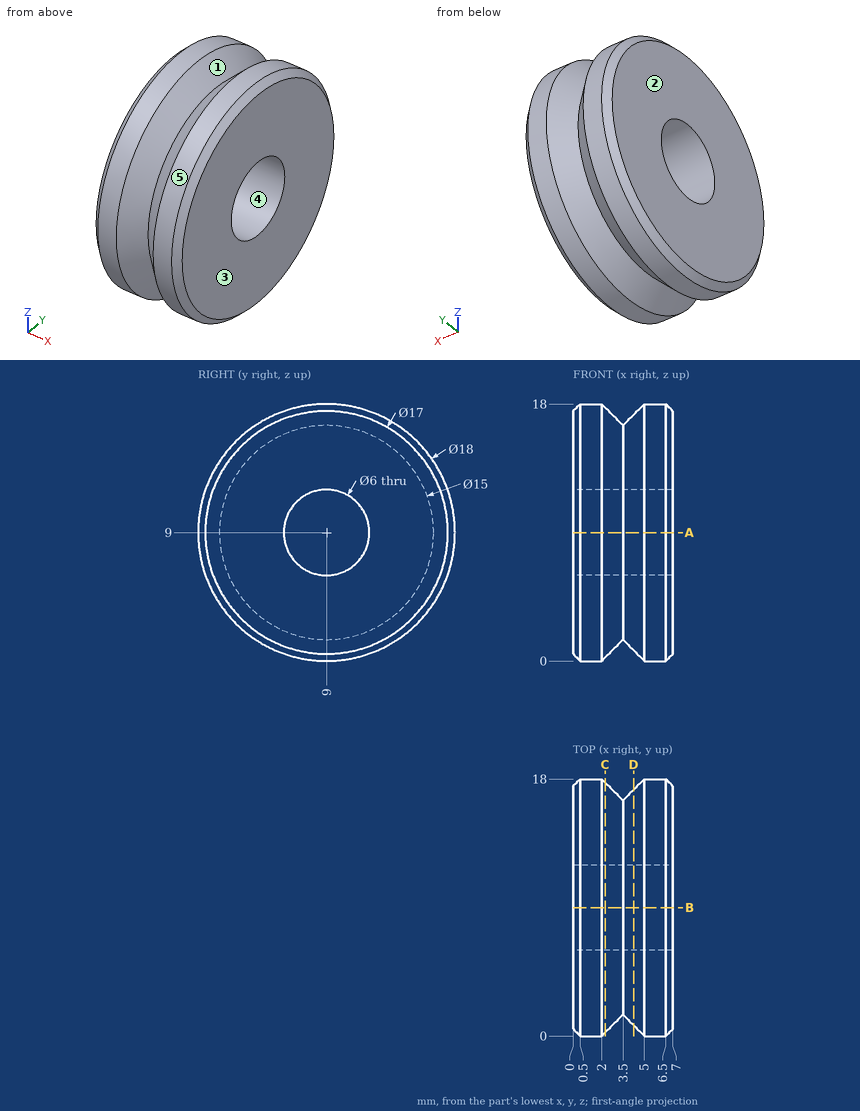
Print and shaded views of the part. All mm, measured from the part's lowest x, y and z. A direction names the side the tool comes from. Coordinates: 2 decimals unless noted, no trailing zeros. Order: outer loops, then holes, each group sorted by start corner. A loop starts at its lowest first (then second) coordinate and runs counter-clockwise, first axis right, second up.
Item 1: Drop flat-ended pins along their axis: pin 1 Ø3 at (x, y) = (4, 7.5) entering from +Z; pin 2 Ø5.5 at (y, z) = (9, 9) entering from +X; pin 3 Ø1.5 at (x, y) = (3.5, 12) entering from -Z; pin 4 Ø2 at (x, y) = (1, 5.5) entering from +Z. Give the stop position or say it passes through.
Filled in:
pin 1: stops at z = 17.99
pin 2: passes through
pin 3: stops at z = 1.27
pin 4: stops at z = 17.65
Item 2: Saw through at D-D on x = 4.25. List the corners of the cut face in (y, z), then the cut area to 3 significant figures.
Filled in:
outline: circle Ø16.5 at (9, 9); hole circle Ø6 at (9, 9)
area: 186 mm2
Item 3: Tool access for the marked faces 1 and 2: list every direction of +Z, -Z, +X, -X, +Y, -Y with a clear straight run to the whole face (end or side of a thin tool).
Filled in:
face 1: none
face 2: +Z, -Z, -X, +Y, -Y
Item 4: Saw through at C-C on x = 2.25. List the corners of the cut face in (y, z).
Filled in:
outline: circle Ø17.5 at (9, 9); hole circle Ø6 at (9, 9)
Item 5: Mould opens along Y. For the marked faces 3, 4 and 5 say: released by +Y, released by -Y, zero draft, split by the parting line, or undercut.
Filled in:
face 3: zero draft
face 4: undercut
face 5: split by the parting line
Item 6: Drill centre lines: L1, parallel to X at y = 11.75, z = 17.25; L2, parallel to Y at x = 3.75, z = 10; L3, parallel to X at y = 13.5, z = 1.5. Where is each one in solid material? Low to high.
Filled in:
L1: x = 0.2 to 2.3, 4.7 to 6.8
L2: y = 1.31 to 6.17, 11.83 to 16.69
L3: x = 0.25 to 2.25, 4.75 to 6.75
Item 7: Saw through at A-A on z = 9. List the corners of the cut face in (x, y).
Filled in:
outline: (0, 0.5) - (0.5, 0) - (2, 0) - (3.5, 1.5) - (5, 0) - (6.5, 0) - (7, 0.5) - (7, 6) - (0, 6) - close; (0, 12) - (7, 12) - (7, 17.5) - (6.5, 18) - (5, 18) - (3.5, 16.5) - (2, 18) - (0.5, 18) - (0, 17.5) - close
